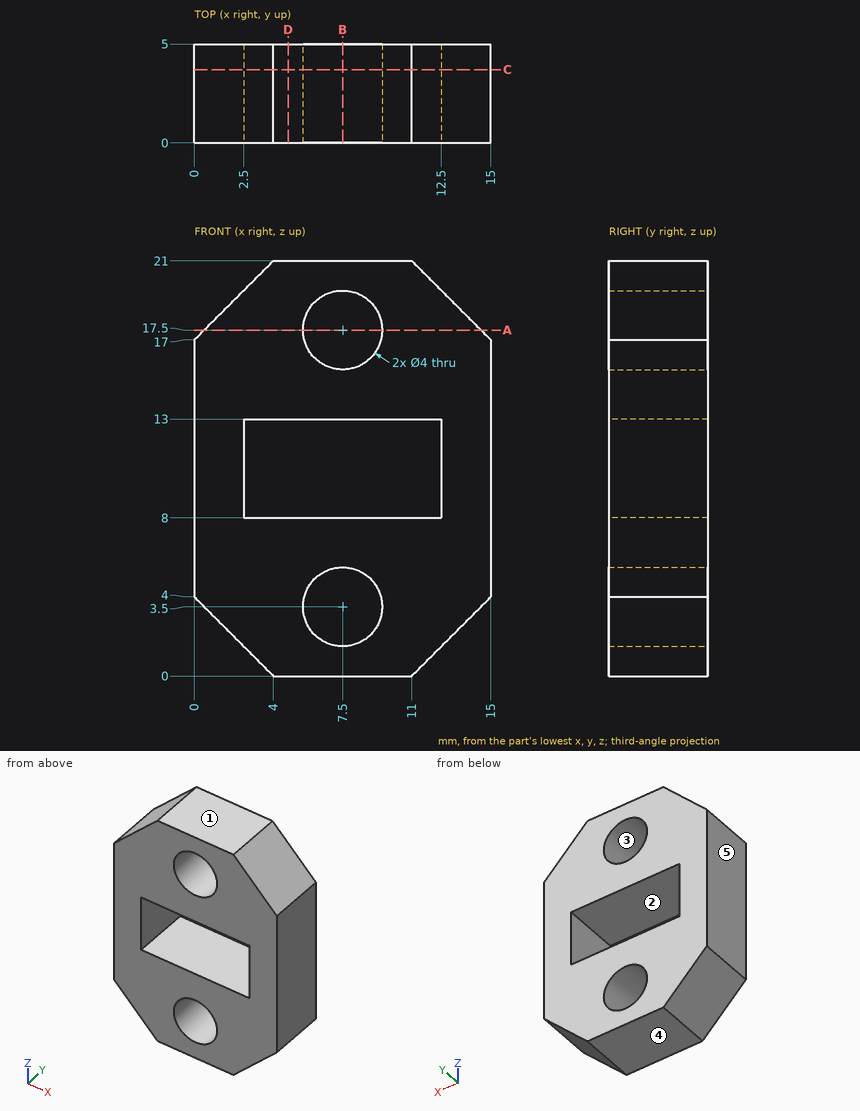
Input: dimensioned drawing with shaded views. Units: mm. Origin: part minimum x, y, z. A direction names the side the tool comes from. Coordinates: 2 decimals unless noted, no trailing zeros. Write each loop counter-clockwise with the first axis right and the second up, starting at its lowest first coordinate (ties: lowest second). Pieces come first, ordered by that corner, then holes. Notation, with made-up numbers: M -14.5,48 L -5.5,48 A26 cw -5.5,83 Z; hole C 41.25,80.5 d3. An arc over 180 degrees is marked long. Use one line per item in the form item = value.
Q1. Section B-B (x = 7.5). Return loops of the section in (y, z).
Answer below:
outline = M 0,0 L 5,0 L 5,1.5 L 0,1.5 Z; M 0,5.5 L 5,5.5 L 5,8 L 0,8 Z; M 0,13 L 5,13 L 5,15.5 L 0,15.5 Z; M 0,19.5 L 5,19.5 L 5,21 L 0,21 Z
Q2. Section D-D (x = 4.75). Return loops of the section in (y, z).
Answer below:
outline = M 0,0 L 5,0 L 5,8 L 0,8 Z; M 0,13 L 5,13 L 5,21 L 0,21 Z
Q3. Material intervals for probe 1 along Z at (x, y) = (7.5, 3.75); probe 2 along Z at (x, y) = (8, 2.9); probe 3 along Z at (x, y) = (10.75, 4.4), sorted ascending. Write a range as from..to.
Answer below:
probe_1 = 0..1.5, 5.5..8, 13..15.5, 19.5..21
probe_2 = 0..1.56, 5.44..8, 13..15.56, 19.44..21
probe_3 = 0..8, 13..21
Q4. Set-up query: the marked faces 1 and 2. Return all of +Z, -Z, +X, -X, +Y, -Y with unobstructed straight access to the full face (end or side cutting, diameter ignored); none if empty.
Answer below:
face_1 = +Z, +X, -X, +Y, -Y
face_2 = +Y, -Y
Q5. Section A-A (z = 17.5). Return loops of the section in (x, y), plus the area to 3 significant figures.
Answer below:
outline = M 0.5,0 L 5.5,0 L 5.5,5 L 0.5,5 Z; M 9.5,0 L 14.5,0 L 14.5,5 L 9.5,5 Z
area = 50.0 mm²
Q6. Section C-C (y = 3.7). Return loops of the section in (x, z).
Answer below:
outline = M 0,4 L 4,0 L 11,0 L 15,4 L 15,17 L 11,21 L 4,21 L 0,17 Z; hole M 2.5,8 L 12.5,8 L 12.5,13 L 2.5,13 Z; hole C 7.5,3.5 d4; hole C 7.5,17.5 d4
Q7. Draft query along Z for the marked faces 3, 4 and 5. Return one class per face: released by +Z, released by -Z, zero draft, split by the parting line, or undercut.
Answer below:
face_3 = undercut
face_4 = released by -Z
face_5 = zero draft
